Part model, mm, in its own coordinate system. Give positions to 0.01 mm unless a question says otherwise; leave off trailing zeros. Order: outer loops, then holes, each group sorted by start corner. A loop starts at its lowest first (then second) coordinate and runs counter-clockwise, first axis right, second up. Notation, with made-up numbers: (46.25, 27.5) -> (104.25, 27.5) arc R20 ccw to (104.25, 40.5) -> close; hole circle Ø4 at (-28, 79). An arc over 180 degrees is marked (long way). Write item = value, one per line. Start each with the question number.
Item 1: Flat gauge pins, fed straight in: P1, Ø0.9, axis at y = -26.5, z = 3.5, coming from the +X side; P2, Ø1.5, axis at x = 27.5, z = 2.5, coming from the -Y side; P3, Ø1.5, axis at x = -21.5, z = 2.5, coming from the +Y side. Where does each tip first touch, or does it go through?
Item 2: Band-saw the part on C-C on x = 27.5. Write the cut outline in (y, z), plus the area to 3 significant figures.
Item 3: Band-saw the part on B-B on x = -21. Write the cut outline in (y, z).
Item 4: Drill centre lines: line 1 along X through (y, z) = (32, 2.5); line 2 along X through (y, z) = (-20.5, 2); line 3 along Y through (x, z) = (21, 3.5). Where is each one in solid material? Low to high.
Item 5: Band-saw the part on A-A on y = -23.5. Write the cut outline in (x, z), plus the area to 3 significant figures.
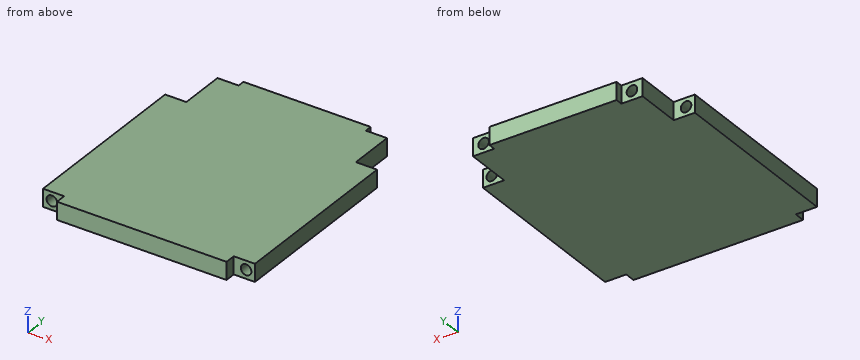
```python
from build123d import *

# Parameters (mm, degrees)
EXTRUDE_1_DEPTH     = 5
SKETCH_2_R          = 1.5
CUT_EXTRUDE_1_DEPTH = 10
SKETCH_3_R          = 1.5
CUT_EXTRUDE_2_DEPTH = 10


with BuildPart() as part:
    # ｽｹｯﾁ1 → ﾎﾞｽ - 押し出し1 (new body)
    with BuildSketch(Plane.XY):
        Polygon((30, -25.5), (30, 25.5), (24, 25.5), (24, 38.5), (18, 38.5), (18, 40.5), (-18, 40.5), (-18, 38.5), (-24, 38.5), (-24, 25.5), (-30, 25.5), (-30, -25.5), (-24, -25.5), (-24, -28.5), (24, -28.5), (24, -25.5), align=None)
    extrude(amount=EXTRUDE_1_DEPTH)

    # ｽｹｯﾁ2 → ｶｯﾄ - 押し出し1 (cut)
    with BuildSketch(Plane(origin=(0, 25.5, 0), x_dir=(1, 0, 0), z_dir=(0, 1, 0))):
        with Locations(Location((-27.5, -2.5, 0), (0, 0, 180))):
            Circle(SKETCH_2_R)
        with Locations((27.5, -2.5)):
            Circle(SKETCH_2_R)
    cut_extrude_1 = extrude(amount=-CUT_EXTRUDE_1_DEPTH, mode=Mode.SUBTRACT)

    # ﾐﾗｰ1: ｶｯﾄ - 押し出し1 across plane
    add(cut_extrude_1.mirror(Plane.ZX), mode=Mode.SUBTRACT)

    # ｽｹｯﾁ3 → ｶｯﾄ - 押し出し2 (cut)
    with BuildSketch(Plane(origin=(0, 38.5, 0), x_dir=(1, 0, 0), z_dir=(0, 1, 0))):
        with Locations(Location((-21, -2.5, 0), (0, 0, 270))):
            Circle(SKETCH_3_R)
        with Locations(Location((21, -2.5, 0), (0, 0, 90))):
            Circle(SKETCH_3_R)
    extrude(amount=-CUT_EXTRUDE_2_DEPTH, mode=Mode.SUBTRACT)


solid = part.part
```
Values found:
q1.P1 = 24
q1.P2 = -15.5
q1.P3 = 28.5
q2.outline = (-25.5, 0) -> (25.5, 0) -> (25.5, 1) -> (15.5, 1) -> (15.5, 4) -> (25.5, 4) -> (25.5, 5) -> (-25.5, 5) -> (-25.5, 4) -> (-15.5, 4) -> (-15.5, 1) -> (-25.5, 1) -> close
q2.area = 195 mm^2
q3.outline = (-28.5, 0) -> (38.5, 0) -> (38.5, 1) -> (28.5, 1) -> (28.5, 4) -> (38.5, 4) -> (38.5, 5) -> (-28.5, 5) -> close
q4.line_1 = -24 to -22.5, -19.5 to 19.5, 22.5 to 24
q4.line_2 = -30 to -28.91, -26.09 to 26.09, 28.91 to 30
q4.line_3 = -28.5 to 28.5
q5.outline = (-30, 0) -> (30, 0) -> (30, 5) -> (-30, 5) -> close; hole circle Ø3 at (-27.5, 2.5); hole circle Ø3 at (27.5, 2.5)
q5.area = 286 mm^2
